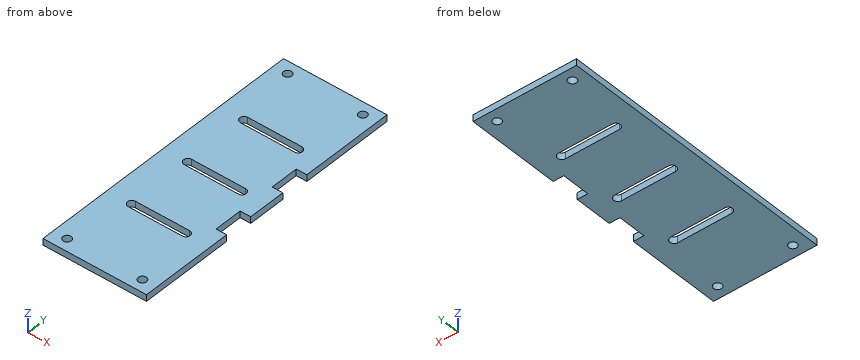
from build123d import *

# Parameters (mm, degrees)
COVER_WITH_CLAMP_HARDWARE_CLEARANCES_PRO_R = 1.75
COVER_WITH_CLAMP_HARDWARE_CLEARANCES_DEPTH = 2.8


with BuildPart() as part:
    # Cover with clamp hardware clearances profile → Cover with clamp hardware clearances (new body)
    with BuildSketch(Plane.XY):
        Polygon((-22, -60), (22, -60), (22, -20), (17.5, -20), (17.5, -8), (22, -8), (22, 8), (17.5, 8), (17.5, 20), (22, 20), (22, 60), (-22, 60), align=None)
        with Locations((-16, -55)):
            Circle(COVER_WITH_CLAMP_HARDWARE_CLEARANCES_PRO_R, mode=Mode.SUBTRACT)
        with Locations((-16, 55)):
            Circle(COVER_WITH_CLAMP_HARDWARE_CLEARANCES_PRO_R, mode=Mode.SUBTRACT)
        with Locations((16, -55)):
            Circle(COVER_WITH_CLAMP_HARDWARE_CLEARANCES_PRO_R, mode=Mode.SUBTRACT)
        with Locations((16, 55)):
            Circle(COVER_WITH_CLAMP_HARDWARE_CLEARANCES_PRO_R, mode=Mode.SUBTRACT)
        with BuildLine():
            Line((-11.5, -29.8), (11.5, -29.8))
            ThreePointArc((11.5, -29.8), (13.3, -28), (11.5, -26.2))
            Line((11.5, -26.2), (-11.5, -26.2))
            ThreePointArc((-11.5, -26.2), (-13.3, -28), (-11.5, -29.8))
        make_face(mode=Mode.SUBTRACT)
        with BuildLine():
            Line((-11.5, -1.8), (11.5, -1.8))
            ThreePointArc((11.5, -1.8), (13.3, 0), (11.5, 1.8))
            Line((11.5, 1.8), (-11.5, 1.8))
            ThreePointArc((-11.5, 1.8), (-13.3, 0), (-11.5, -1.8))
        make_face(mode=Mode.SUBTRACT)
        with BuildLine():
            Line((-11.5, 26.2), (11.5, 26.2))
            ThreePointArc((11.5, 26.2), (13.3, 28), (11.5, 29.8))
            Line((11.5, 29.8), (-11.5, 29.8))
            ThreePointArc((-11.5, 29.8), (-13.3, 28), (-11.5, 26.2))
        make_face(mode=Mode.SUBTRACT)
    extrude(amount=COVER_WITH_CLAMP_HARDWARE_CLEARANCES_DEPTH)


solid = part.part
Geometry: final body of the model. Coordinates: model frame, mm. Coordinates: 2 decimals unless noted, no trailing zeros. Loops run counter-clockwise (first coordinate to the right, second up) from the corner with the lowest first, then second, coordinate; pieces in that order, holes last. Notation, with made-up numbers: (8, -0.75) - (66, -0.75) arc R10 ccw to (66, 15.25) - close; hole circle Ø8 at (67, 61). An arc over 180 degrees is marked (long way). Put each result on its own line as item: value. Start each with the question number.
Q1. Line query: line 1 (Y direction, x = 16, z = 0.9); line 2 (Y direction, x = -8.5, z = 0.8); line 3 (Y direction, x = 19, z = 1.6). Output: solid intervals per line, ascending.
Q2. Cut plane A-A, the plane x = 4. Return loops of the section in (y, z).
Q3. Pin query (flat end, axial travel): pin 1 Ø1.4 at (y, z) = (-14, 2) entering from +X. Return the tip coordinate at first contact, or that it passes through.
Q4. Cut plane C-C, the plane z = 1.75. Return loops of the section in (x, y), and give its area (3 significant figures).
Q5. Cut plane D-D, the plane y = -28. Return loops of the section in (x, z), and give its area (3 significant figures).
Q6. Cut plane B-B, the plane y = 55. Return loops of the section in (x, z), and give its area (3 significant figures).
Filled sheet:
1. line 1: -60 to -56.75, -53.25 to 53.25, 56.75 to 60
1. line 2: -60 to -29.8, -26.2 to -1.8, 1.8 to 26.2, 29.8 to 60
1. line 3: -60 to -20, -8 to 8, 20 to 60
2. outline: (-60, 0) - (-29.8, 0) - (-29.8, 2.8) - (-60, 2.8) - close; (-26.2, 0) - (-1.8, 0) - (-1.8, 2.8) - (-26.2, 2.8) - close; (1.8, 0) - (26.2, 0) - (26.2, 2.8) - (1.8, 2.8) - close; (29.8, 0) - (60, 0) - (60, 2.8) - (29.8, 2.8) - close
3. pin 1: x = 17.5
4. outline: (-22, -60) - (22, -60) - (22, -20) - (17.5, -20) - (17.5, -8) - (22, -8) - (22, 8) - (17.5, 8) - (17.5, 20) - (22, 20) - (22, 60) - (-22, 60) - close; hole circle Ø3.5 at (-16, -55); hole circle Ø3.5 at (-16, 55); hole (-11.5, -29.8) - (11.5, -29.8) arc R1.8 ccw to (11.5, -26.2) - (-11.5, -26.2) arc R1.8 ccw to start; hole (-11.5, -1.8) - (11.5, -1.8) arc R1.8 ccw to (11.5, 1.8) - (-11.5, 1.8) arc R1.8 ccw to start; hole (-11.5, 26.2) - (11.5, 26.2) arc R1.8 ccw to (11.5, 29.8) - (-11.5, 29.8) arc R1.8 ccw to start; hole circle Ø3.5 at (16, -55); hole circle Ø3.5 at (16, 55)
4. area: 4,850 mm²
5. outline: (-22, 0) - (-13.3, 0) - (-13.3, 2.8) - (-22, 2.8) - close; (13.3, 0) - (22, 0) - (22, 2.8) - (13.3, 2.8) - close
5. area: 48.7 mm²
6. outline: (-22, 0) - (-17.75, 0) - (-17.75, 2.8) - (-22, 2.8) - close; (-14.25, 0) - (14.25, 0) - (14.25, 2.8) - (-14.25, 2.8) - close; (17.75, 0) - (22, 0) - (22, 2.8) - (17.75, 2.8) - close
6. area: 104 mm²
